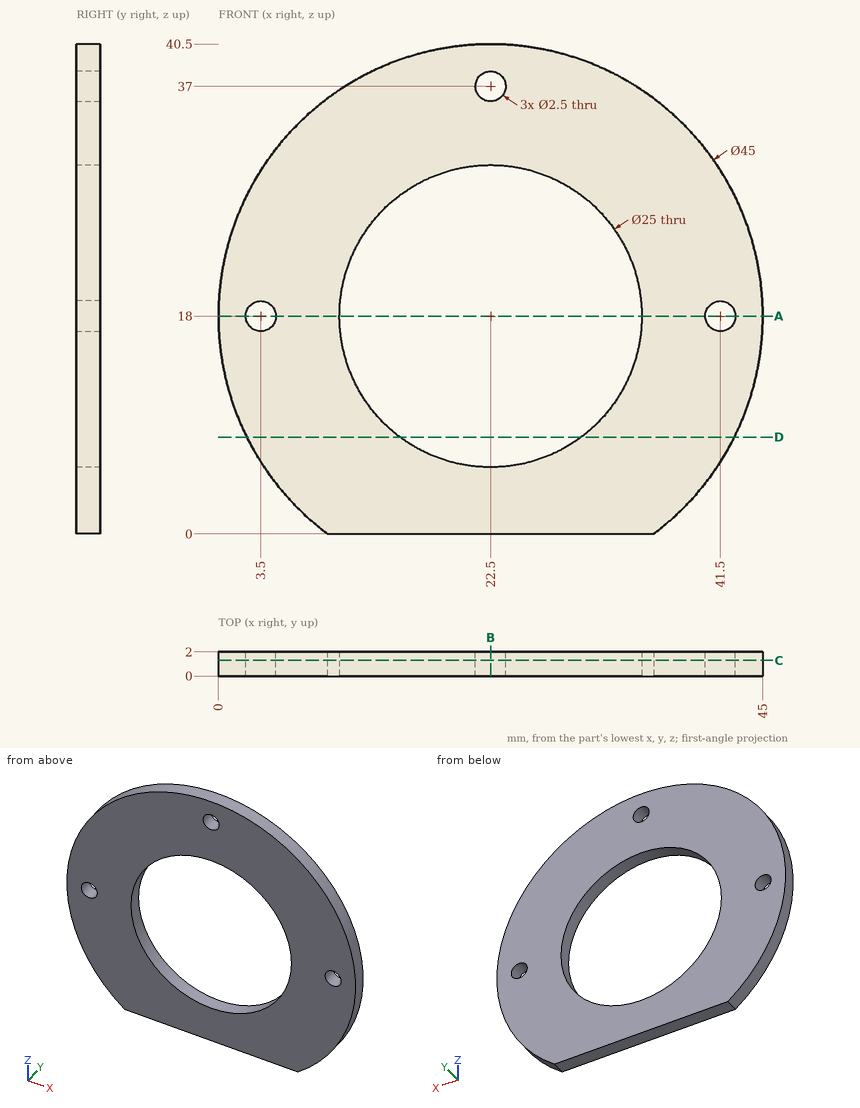
Check sheet for the drawn part. Datum: minimum x, y, z corner. Units: mm. Coordinates: 2 decimals unless noted, no trailing zeros. Order: outer loops, then holes, each group sorted by start corner. A loop starts at its lowest first (then second) coordinate and runs counter-clockwise, first axis right, second up. Notation, with made-up numbers: M 54,15.5 L 89,15.5 A31 ccw 89,49.5 Z; hole C 12.5,66 d1. An arc over 180 degrees is marked long. One line per question, with ' | ' between items. Start each with the question number.
Item 1: Cross-section at B-B on x = 22.5. Enter the section's corners in (y, z), then the cut area to 3 significant figures.
Item 2: Material ranges on L1, parallel to X at y = 0.5, z = 18; L2, parallel to X at y = 1.6, z = 11; L3, parallel to Z at x = 16.5, y = 0.65, recorded low to high. Write a range as [from, to].
Item 3: Cross-section at D-D on z = 8. Enter the section's corners in (x, y).
Item 4: Cross-section at C-C on y = 1.3. Enter the section's corners in (x, z), then the cut area to 3 significant figures.
Item 5: Cross-section at A-A on z = 18. Enter the section's corners in (x, y), then the cut area to 3 significant figures.
Item 6: Gauge pin test, flat ends, axial feed: pin 1 (2 mm diameter, centred on x = 41.5, z = 18, fed in from -Y); pin 2 (1 mm diameter, centred on x = 9, y = 0.5, fed in from +Z). Record the tip position at first contact, or that the pin passes through.
Findings:
1) outline: M 0,0 L 2,0 L 2,5.5 L 0,5.5 Z; M 0,30.5 L 2,30.5 L 2,35.75 L 0,35.75 Z; M 0,38.25 L 2,38.25 L 2,40.5 L 0,40.5 Z | area: 26.0 mm²
2) L1: x = [0, 2.25], [4.75, 10], [35, 40.25], [42.75, 45] | L2: x = [1.12, 12.14], [32.86, 43.88] | L3: z = [0, 7.03], [28.97, 39.69]
3) outline: M 2.34,0 L 15,0 L 15,2 L 2.34,2 Z; M 30,0 L 42.66,0 L 42.66,2 L 30,2 Z
4) outline: M 9,0 L 36,0 A22.5 ccw long Z; hole C 3.5,18 d2.5; hole C 22.5,18 d25; hole C 22.5,37 d2.5; hole C 41.5,18 d2.5 | area: 1,000 mm²
5) outline: M 0,0 L 2.25,0 L 2.25,2 L 0,2 Z; M 4.75,0 L 10,0 L 10,2 L 4.75,2 Z; M 35,0 L 40.25,0 L 40.25,2 L 35,2 Z; M 42.75,0 L 45,0 L 45,2 L 42.75,2 Z | area: 30.0 mm²
6) pin 1: passes through | pin 2: stops at z = 36.36
